```python
from build123d import *

# Parameters (mm, degrees)
SKETCH_1_R          = 1.7
SKETCH_1_R_2        = 1
SKETCH_1_W          = 4
SKETCH_1_H          = 24
SKETCH_1_W_2        = 3
SKETCH_1_H_2        = 3
EXTRUDE_1_DEPTH     = 2
SKETCH_2_W          = 3
SKETCH_2_H          = 3
SKETCH_2_R          = 1.7
EXTRUDE_2_DEPTH     = 6
FILLET_2_R          = 3
SKETCH_4_R          = 2.5
CUT_EXTRUDE_2_DEPTH = 1
SKETCH_5_R          = 2.5
CUT_EXTRUDE_3_DEPTH = 1
CUT_EXTRUDE_4_DEPTH = 10


with BuildPart() as part:
    # 草图1 → 凸台-拉伸1 (new body)
    with BuildSketch(Plane.XY):
        with BuildLine():
            Line((4, 46), (-4, 46))
            ThreePointArc((-4, 46), (-5.984059393, 43.747991415), (-3.5, 42.063508327))
            Line((-3.5, 42.063508327), (-3.5, 42))
            Line((-3.5, 42), (-3.5, 0))
            ThreePointArc((-3.5, 0), (0, -3.5), (3.5, 0))
            Line((3.5, 0), (3.5, 42))
            Line((3.5, 42), (3.5, 42.063508327))
            ThreePointArc((3.5, 42.063508327), (5.984059393, 43.747991415), (4, 46))
        make_face()
        Circle(SKETCH_1_R, mode=Mode.SUBTRACT)
        with Locations((-4, 44)):
            Circle(SKETCH_1_R_2, mode=Mode.SUBTRACT)
        with Locations((4, 44)):
            Circle(SKETCH_1_R_2, mode=Mode.SUBTRACT)
        with Locations((0, 30)):
            Rectangle(SKETCH_1_W, SKETCH_1_H, mode=Mode.SUBTRACT)
        with Locations((0, 12)):
            Rectangle(SKETCH_1_W_2, SKETCH_1_H_2, mode=Mode.SUBTRACT)
    extrude(amount=EXTRUDE_1_DEPTH)

    # 草图2 → 凸台-拉伸2 (add)
    with BuildSketch(Plane(origin=(0, 0, 0), x_dir=(-1, 0, 0), z_dir=(0, 0, -1))):
        Polygon((3.5, 15.5), (-3.5, 15.5), (-3.5, 8.5), (-1, 8.5), (1, 8.5), (3.5, 8.5), align=None)
        with Locations((0, 12)):
            Rectangle(SKETCH_2_W, SKETCH_2_H, mode=Mode.SUBTRACT)
        with BuildLine():
            Line((1, 8.5), (-1, 8.5))
            Line((-1, 8.5), (-1, 3.354101966))
            ThreePointArc((-1, 3.354101966), (0, 3.5), (1, 3.354101966))
            Line((1, 3.354101966), (1, 8.5))
        make_face()
        with BuildLine():
            ThreePointArc((-1, 3.354101966), (-2.80624304, 2.091650066), (-3.5, 0))
            ThreePointArc((-3.5, 0), (0, -3.5), (3.5, 0))
            ThreePointArc((3.5, 0), (2.80624304, 2.091650066), (1, 3.354101966))
            ThreePointArc((1, 3.354101966), (0, 3.5), (-1, 3.354101966))
        make_face()
        Circle(SKETCH_2_R, mode=Mode.SUBTRACT)
    extrude(amount=EXTRUDE_2_DEPTH)

    # 圆角2
    fillet_2_edges = [part.edges().sort_by_distance(p)[0] for p in [
        (3.5, 42.063508327, 1),
        (-3.5, 42.063508327, 1),
    ]]
    fillet(fillet_2_edges, radius=FILLET_2_R)

    # 草图4 → 切除-拉伸2 (cut)
    with BuildSketch(Plane.XY.offset(2)):
        Circle(SKETCH_4_R)
    extrude(amount=-CUT_EXTRUDE_2_DEPTH, mode=Mode.SUBTRACT)

    # 草图5 → 切除-拉伸3 (cut)
    with BuildSketch(Plane(origin=(0, 0, -6), x_dir=(-1, 0, 0), z_dir=(0, 0, -1))):
        Circle(SKETCH_5_R)
    extrude(amount=-CUT_EXTRUDE_3_DEPTH, mode=Mode.SUBTRACT)

    # 草图3 → 切除-拉伸4 (cut)
    with BuildSketch(Plane.XY.offset(2)):
        with BuildLine():
            Line((-5.366025404, 44.5), (-5.366025404, 43.5))
            Line((-5.366025404, 43.5), (-4.866025404, 43.5))
            ThreePointArc((-4.866025404, 43.5), (-5, 44), (-4.866025404, 44.5))
            Line((-4.866025404, 44.5), (-5.366025404, 44.5))
        make_face()
        with BuildLine():
            ThreePointArc((-5.936491673, 44.5), (-6, 44), (-5.936491673, 43.5))
            Line((-5.936491673, 43.5), (-5.366025404, 43.5))
            Line((-5.366025404, 43.5), (-5.366025404, 44.5))
            Line((-5.366025404, 44.5), (-5.936491673, 44.5))
        make_face()
        with BuildLine():
            ThreePointArc((-5.366025404, 45.460812992), (-5.719722408, 45.021055747), (-5.936491673, 44.5))
            Line((-5.936491673, 44.5), (-5.366025404, 44.5))
            Line((-5.366025404, 44.5), (-5.366025404, 45.460812992))
        make_face()
        with BuildLine():
            Line((-5.366025404, 43.5), (-5.936491673, 43.5))
            ThreePointArc((-5.936491673, 43.5), (-5.719722408, 42.978944253), (-5.366025404, 42.539187008))
            Line((-5.366025404, 42.539187008), (-5.366025404, 43.5))
        make_face()
        with BuildLine():
            ThreePointArc((5.936491673, 43.5), (6, 44), (5.936491673, 44.5))
            Line((5.936491673, 44.5), (5.366025404, 44.5))
            Line((5.366025404, 44.5), (5.366025404, 43.5))
            Line((5.366025404, 43.5), (5.936491673, 43.5))
        make_face()
        with BuildLine():
            Line((5.366025404, 44.5), (5.936491673, 44.5))
            ThreePointArc((5.936491673, 44.5), (5.719722408, 45.021055747), (5.366025404, 45.460812992))
            Line((5.366025404, 45.460812992), (5.366025404, 44.5))
        make_face()
        with BuildLine():
            Line((5.366025404, 43.5), (5.366025404, 44.5))
            Line((5.366025404, 44.5), (4.866025404, 44.5))
            ThreePointArc((4.866025404, 44.5), (4.965925826, 44.258819045), (5, 44))
            ThreePointArc((5, 44), (4.965925826, 43.741180955), (4.866025404, 43.5))
            Line((4.866025404, 43.5), (5.366025404, 43.5))
        make_face()
        with BuildLine():
            ThreePointArc((5.366025404, 42.539187008), (5.719722408, 42.978944253), (5.936491673, 43.5))
            Line((5.936491673, 43.5), (5.366025404, 43.5))
            Line((5.366025404, 43.5), (5.366025404, 42.539187008))
        make_face()
    extrude(amount=-CUT_EXTRUDE_4_DEPTH, mode=Mode.SUBTRACT)


solid = part.part
```
CAD build for the part. Positions are in the model's coordinates, mm. A direction names the side the tool comes from. Round coordinates to 2 decimals unless told otherwise and drop trailing zeros. Write each loop counter-clockwise with the first axis right and the second up, starting at its lowest first coordinate (ties: lowest second). Pieces come first, ordered by that corner, then holes. Notation, with made-up numbers: (28.25, -22) -> (69.25, -22) arc R14 ccw to (69.25, -9) -> close; hole circle Ø4 at (20, 65.5). An arc over 180 degrees is marked (long way). Answer in a Markdown table with one row per item. Add a question column.
Item 1: Mould opens along X. For faces 1 (the face through (2, -1, 1)), 2 (the face through (-5.366, 45, 1)), 3 (the face through (-2, 5, 0)) say: pulls with the +X half, pulls with the -X half, needs draft (parallel to the pull), parting line crosses it, or undercut.
Item 2: Saw through at C-C, the plane z = 0.5. Count the separate pieces of the cut face and the enclosed holes in it, then the cut area to 3 significant figures.
Item 3: Which spindle directions (+Z, -Z, +X, -X, +Y, -Y) get a long thin tool onto all of the face, cutting with end or side? Do faces 4 (the face through (0, 18, 1)), 5 (the face through (0.54, -2.44, -5.51)), 6 (the face through (-3.5, 15, 0)). Say none if no direction does.
Item 4: Saw through at B-B, the plane y = 35. Write the cut outline in (x, z).
Item 5: Drill centre lines: line 1 (Y direction, x = 0, z = 1.25); line 2 (Y direction, x = 0, z = -5.65); line 3 (Y direction, x = 0.5, z = 1.75). Where is each one in solid material? Low to high. Write a range as from..to.
Item 6: Saw through at A-A, the plane x = 0. Write the cut outline in (y, z), then the cut area to 3 significant figures.
Item 7: Drop flat-ended pins along their axis: pin 1 Ø1.2 at (x, y) = (4, 44) entering from -Z; pin 2 Ø3 at (x, z) = (2, -4.5) entering from -Y; pin 3 Ø4.5 at (x, y) = (0, 0) entering from +Z; pin 4 Ø3.5 at (y, z) = (11.5, -2) entering from -X. Give the stop position or say it passes through.
Item 8: Saw through at D-D, the plane y = 4. Write the cut outline in (x, z), then the cut area to 3 significant figures.
Findings below:
| question | item | result |
|---|---|---|
| 1 | face 1 | undercut |
| 1 | face 2 | pulls with the -X half |
| 1 | face 3 | needs draft |
| 2 | separate pieces | 1 |
| 2 | enclosed holes | 3 |
| 2 | area | 236 mm^2 |
| 3 | face 4 | +Z, -Z |
| 3 | face 5 | -Z |
| 3 | face 6 | +Z, -Z, -X, -Y |
| 4 | outline | (-3.5, 0) -> (-2, 0) -> (-2, 2) -> (-3.5, 2) -> close; (2, 0) -> (3.5, 0) -> (3.5, 2) -> (2, 2) -> close |
| 5 | line 1 | y = -3.5..-2.5, 2.5..10.5, 13.5..18, 42..46 |
| 5 | line 2 | y = -3.5..-2.5, 2.5..10.5, 13.5..15.5 |
| 5 | line 3 | y = -3.46..-2.45, 2.45..10.5, 13.5..18, 42..46 |
| 6 | outline | (-3.5, -6) -> (-2.5, -6) -> (-2.5, -5) -> (-1.7, -5) -> (-1.7, 1) -> (-2.5, 1) -> (-2.5, 2) -> (-3.5, 2) -> close; (1.7, -5) -> (2.5, -5) -> (2.5, -6) -> (10.5, -6) -> (10.5, 2) -> (2.5, 2) -> (2.5, 1) -> (1.7, 1) -> close; (13.5, -6) -> (15.5, -6) -> (15.5, 0) -> (18, 0) -> (18, 2) -> (13.5, 2) -> close; (42, 0) -> (46, 0) -> (46, 2) -> (42, 2) -> close |
| 6 | area | 111 mm^2 |
| 7 | pin 1 | passes through |
| 7 | pin 2 | stops at y = -3.46 |
| 7 | pin 3 | stops at z = 1 |
| 7 | pin 4 | stops at x = -3.5 |
| 8 | outline | (-3.5, 0) -> (-1, 0) -> (-1, -6) -> (1, -6) -> (1, 0) -> (3.5, 0) -> (3.5, 2) -> (-3.5, 2) -> close |
| 8 | area | 26.0 mm^2 |
